Part print with two shaded views. Sizes in mm from the minimum x, y, z corner. A direction names the side the tool comes from. Coordinates: 2 decimals unless noted, no trailing zeros. Loops run counter-clockwise (first coordinate to the right, second up) from the corner with the lowest first, then second, coordinate; pieces in that order, holes last.
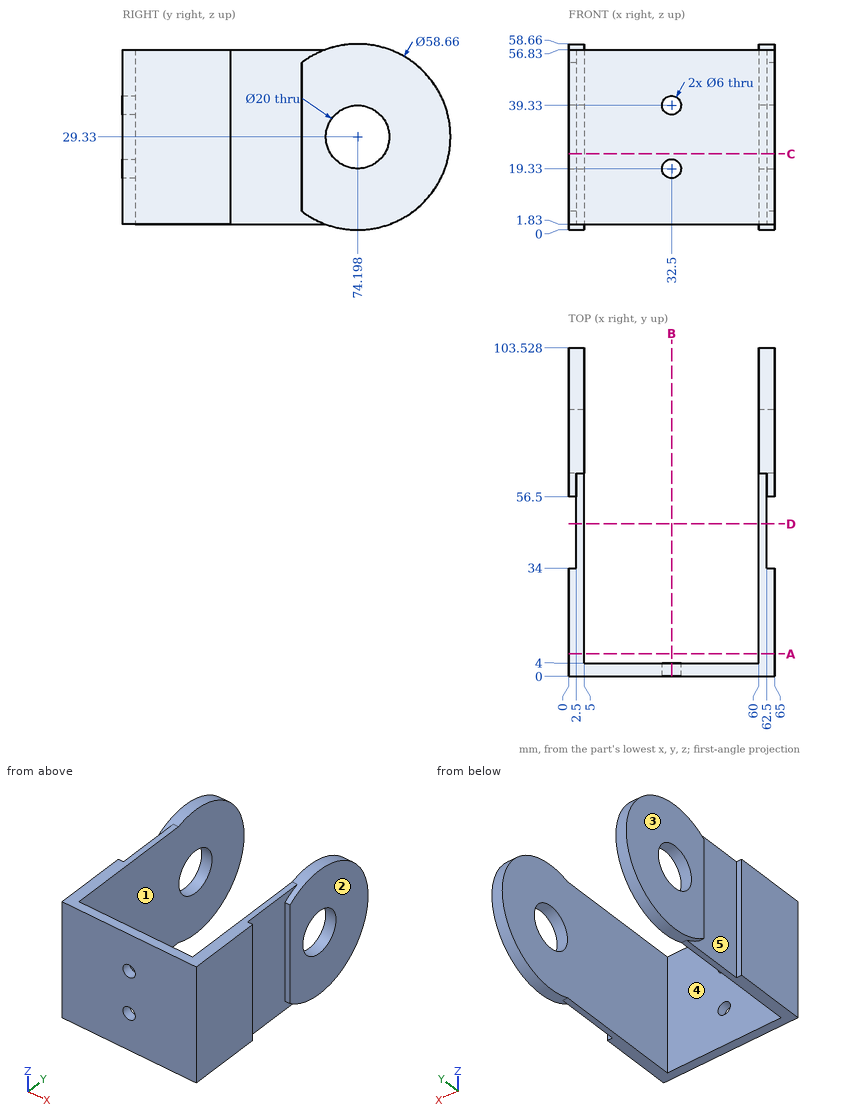
Q1. Drill centre lines: line 1 (X direction, y = 33, z = 20); line 2 (X direction, y = 51.5, z = 18.5); line 3 (Z direction, x = 32.5, y = 3.15). Where is each one in solid material? Low to high.
Answers:
line 1: x = 0 to 5, 60 to 65
line 2: x = 2.5 to 5, 60 to 62.5
line 3: z = 1.83 to 16.33, 22.33 to 36.33, 42.33 to 56.83
Q2. Flat gauge pins, fed straight in: P1, Ø3, axis at x = 33.5, z = 26, coming from the +Y side; P2, Ø16, axis at y = 74.2, z = 29.33, coming from the +X side; P3, Ø1.2, axis at x = 63.5, z = 34, coming from the +Y side; P4, Ø15, axis at y = 46, z = 17, coming from the +X side. Where does each tip first touch, or does it go through?
Answers:
P1: stops at y = 4
P2: passes through
P3: stops at y = 103.24
P4: stops at x = 62.5
Q3. Slice it at B-B (x = 32.5). List the corners of the cut face in (y, z).
Answers:
outline: (0, 1.83) - (4, 1.83) - (4, 16.33) - (0, 16.33) - close; (0, 22.33) - (4, 22.33) - (4, 36.33) - (0, 36.33) - close; (0, 42.33) - (4, 42.33) - (4, 56.83) - (0, 56.83) - close
Q4. Slice it at C-C (z = 24). List the corners of the cut face in (x, y).
Answers:
outline: (0, 0) - (65, 0) - (65, 34) - (62.5, 34) - (62.5, 56.5) - (65, 56.5) - (65, 65.74) - (60, 65.74) - (60, 4) - (5, 4) - (5, 65.74) - (0, 65.74) - (0, 56.5) - (2.5, 56.5) - (2.5, 34) - (0, 34) - close; (0, 82.66) - (5, 82.66) - (5, 103.04) - (0, 103.04) - close; (60, 82.66) - (65, 82.66) - (65, 103.04) - (60, 103.04) - close
Q5. Slice it at A-A (y = 7). List the corners of the cut face in (x, z).
Answers:
outline: (0, 1.83) - (5, 1.83) - (5, 56.83) - (0, 56.83) - close; (60, 1.83) - (65, 1.83) - (65, 56.83) - (60, 56.83) - close
Q6. Which spindle directions (+Z, -Z, +X, -X, +Y, -Y) get a long thin tool onto all of the face, cutting with end or side? Do the marked faces 1 and 2. Say none if no direction does.
Answers:
face 1: +Z, -Z, +Y
face 2: +Z, -Z, +X, +Y, -Y
Q7. Mould opens along Y. For the marked faces 3, 4 and 5 say: +Y half, -Y half, draft (parallel to the pull), parting line (faces both ways), or undercut.
Answers:
face 3: draft
face 4: +Y half
face 5: undercut
Q8. Slice it at D-D (y = 48). List the corners of the cut face in (x, z), and give its area (3 significant figures).
Answers:
outline: (2.5, 1.83) - (5, 1.83) - (5, 56.83) - (2.5, 56.83) - close; (60, 1.83) - (62.5, 1.83) - (62.5, 56.83) - (60, 56.83) - close
area: 275 mm2
